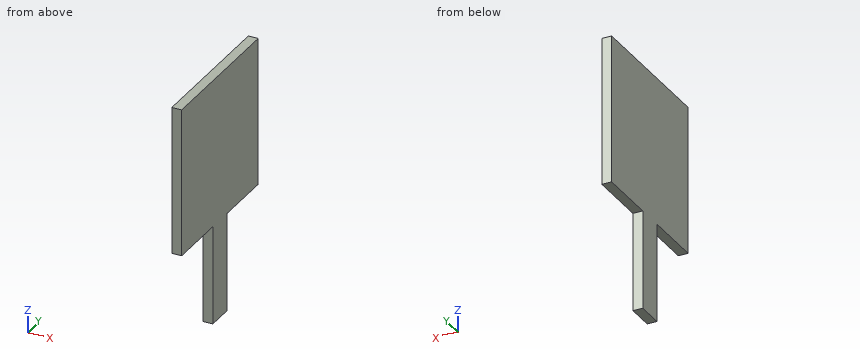
from build123d import *

# Parameters (mm, degrees)
F1_DEPTH = 1


# Not quite as in the source:
# - a feature names something its author has since deleted; it is built from what else it names


with BuildPart() as f1:
    # F0 (on Right) → F1 (new body)
    with BuildSketch(Plane.YZ):
        Polygon((11.5, 0), (0, 0), (-1.75, 0), (-1.75, -15), (0, -15), (4.35, -15), (4.35, -25), (5.25, -25), (6.25, -25), (7.15, -25), (7.15, -15), (11.5, -15), (13.25, -15), (13.25, 0), align=None)
    extrude(amount=F1_DEPTH)


solid = f1.part
Geometry check sheet. Reference: the model listing, model coordinates, mm. Give positions to 0.01 mm unless a question says otherwise; leave off trailing zeros. Order: outer loops, then holes, each group sorted by start corner. A loop starts at its lowest first (then second) coordinate and runs counter-clockwise, first axis right, second up. Notation, with made-up numbers: M 78,89.25 L 104,89.25 A17 ccw 104,100.25 Z; hole C -17.5,65 d9. An arc over 180 degrees is marked long. Use a Markdown table: item, result.
Item 1: Section check A-A (x = 0.45). Record the cut outline in (y, z).
Answers follow:
| item | result |
|---|---|
| outline | M -1.75,-15 L 4.35,-15 L 4.35,-25 L 7.15,-25 L 7.15,-15 L 13.25,-15 L 13.25,0 L -1.75,0 Z |
Item 2: Material ranges on line 1 along Z through (x, y) = (0.2, 8.25); line 2 along Y through (x, z) = (0.8, -23.5), recorded low to high.
Answers follow:
| item | result |
|---|---|
| line 1 | z = -15 to 0 |
| line 2 | y = 4.35 to 7.15 |
Item 3: Section check B-B (z = -20.75). Record the cut outline in (x, y).
Answers follow:
| item | result |
|---|---|
| outline | M 0,4.35 L 1,4.35 L 1,7.15 L 0,7.15 Z |
Item 4: Section check C-C (y = 8). Record the cut outline in (x, z).
Answers follow:
| item | result |
|---|---|
| outline | M 0,-15 L 1,-15 L 1,0 L 0,0 Z |
